For this review, take the finished solid that the model builds, in its own axes (mm). Face numbers are marked on the shaded views. Coordinates: 2 decimals unless noted, no trailing zeros. Write each loop counter-clockwise with the first axis right and the second up, starting at its lowest first coordinate (ties: lowest second). Pieces come first, ordered by that corner, then holes. Notation, with made-up numbers: (77, 75) - (107, 75) arc R27 cw to (107, 111) - close; hole circle Ø10 at (19.25, 68.25). An arc over 180 degrees is marked (long way). Use one line per item in the form item = value. Start each with the question number.
1) Mouldability with a two-part tool opening along X and no side actions: class the marked faces 1 and 2 as pulls with the +X half, pulls with the -X half, needs draft (parallel to the pull), parting line crosses it, or undercut.
2) Insertion check: P1, Ø1, axis at y = -14.5, z = 17, coming from the -X side; P2, Ø1.5, axis at x = 2, z = 4.5, coming from the +Y side; P3, Ø3, axis at x = -110, y = 18.5, coming from the +Z side. Each pin has a flat end and moves straight along its axis. Give the tip position at first contact, or say it passes through.
3) We need section A-A (z = 20.5). Give the boundary of the cut face in (x, y), plus the area to 3 significant figures.
4) We need section B-B (x = -24). Give the boundary of the cut face in (y, z), plus the area to 3 significant figures.
5) For L1, parallel to Y at x = -130.25, z = 0; L2, parallel to Y at x = -147, z = 0; L3, parallel to X at y = -14.5, z = -16.5, list the stretches that pass through material, from the lowest coordinate up. Write a range as from..to.
```python
from build123d import *

# Parameters (mm, degrees)
BOSS_EXTRUDE1_START      = 80
SKETCH2_R                = 17.5
BOSS_EXTRUDE1_DEPTH      = 80
BOSS_EXTRUDE2_REACH      = 163.943
BOSS_EXTRUDE2_END_RADIUS = 17.5
SKETCH4_R                = 17.5
BOSS_EXTRUDE3_DEPTH      = 5
HOLE1_D                  = 10.106
HOLE1_DEPTH              = 37.5
HOLE1_CBORE_D            = 13
HOLE1_CBORE_DEPTH        = 9.5
HOLE1_TIP                = 2.91735091
CHAMFER1_SIZE            = 2.55
CHAMFER2_SIZE            = 2


with BuildPart() as part:
    # Sketch1 → Revolve1 (revolve)
    with BuildSketch(Plane.XY, mode=Mode.PRIVATE) as revolve1_sk:
        Polygon((-74.5, 22.5), (-74.5, 0), (74.5, 0), (74.5, 22.5), (70, 22.5), (70, 17.5), (-70, 17.5), (-70, 22.5), align=None)
    revolve(revolve1_sk.sketch.rotate(Axis((-74.5, 0, 0), (1, 0, 0)), 270), axis=Axis((-74.5, 0, 0), (1, 0, 0)))

    # Sketch2 → Boss-Extrude1 (add)
    with BuildSketch(Plane.ZY.offset(74.5).offset(BOSS_EXTRUDE1_START)):
        with Locations(Location((0, 0, 0), (0, 0, 180))):
            Circle(SKETCH2_R)
    extrude(amount=-BOSS_EXTRUDE1_DEPTH)

    # Boss-Extrude2: up to this cylinder (the profile starts outside it)
    boss_extrude2_end = Plane(origin=(-114.5, 0, 0), z_dir=(1, 0, 0)) * Cylinder(BOSS_EXTRUDE2_END_RADIUS, 363.886, mode=Mode.PRIVATE)
    # Sketch3 → Boss-Extrude2 (add, up to the surface)
    with BuildSketch(Plane(origin=(0, 20.5, 0), x_dir=(1, 0, 0), z_dir=(0, 1, 0)), mode=Mode.PRIVATE) as boss_extrude2_sk1:
        with BuildLine():
            Line((-134.5, -5), (-94.5, -5))
            ThreePointArc((-94.5, -5), (-89.5, 0), (-94.5, 5))
            Line((-94.5, 5), (-134.5, 5))
            ThreePointArc((-134.5, 5), (-139.5, 0), (-134.5, -5))
        make_face()
    boss_extrude2_tool1 = extrude(boss_extrude2_sk1.sketch, amount=-BOSS_EXTRUDE2_REACH, mode=Mode.PRIVATE) - boss_extrude2_end
    add(boss_extrude2_tool1.solids().sort_by_distance((-114.5, 20.5, 0))[0])

    # Sketch4 → Boss-Extrude3 (add)
    with BuildSketch(Plane(origin=(74.5, 0, 0), x_dir=(0, 0, -1), z_dir=(1, 0, 0))):
        Circle(SKETCH4_R)
    extrude(amount=BOSS_EXTRUDE3_DEPTH)

    # Hole1
    with Locations(Plane.ZY.offset(154.5)):
        with Locations((0, 0)):
            CounterBoreHole(HOLE1_D / 2, HOLE1_CBORE_D / 2, HOLE1_CBORE_DEPTH, depth=HOLE1_DEPTH)
            with Locations((0, 0, -(HOLE1_DEPTH + HOLE1_TIP / 2))):  # 120° drill point
                Cone(0, HOLE1_D / 2, HOLE1_TIP, mode=Mode.SUBTRACT)

    # Chamfer1
    chamfer1_edges = [part.edges().sort_by_distance(p)[0] for p in [
        (-154.5, 0, -6.5),
    ]]
    chamfer(chamfer1_edges, length=CHAMFER1_SIZE)

    # Chamfer2
    chamfer2_edges = [part.edges().sort_by_distance(p)[0] for p in [
        (-154.5, 0, 17.5),
    ]]
    chamfer(chamfer2_edges, length=CHAMFER2_SIZE)


solid = part.part
```
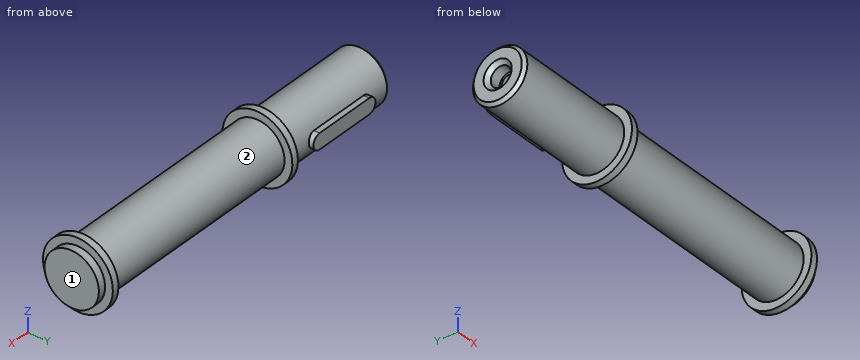
Determined:
q1.face_1 = pulls with the +X half
q1.face_2 = undercut
q2.P1 = -74.5
q2.P2 = 17.09
q2.P3 = 5
q3.outline = (-74.5, -9.27) - (-70, -9.27) - (-70, 9.27) - (-74.5, 9.27) - close; (70, -9.27) - (74.5, -9.27) - (74.5, 9.27) - (70, 9.27) - close
q3.area = 167 mm²
q4.outline = circle Ø35 at (0, 0)
q4.area = 962 mm²
q5.L1 = -17.5..-5.05, 5.05..20.5
q5.L2 = -17.5..-6.5, 6.5..17.5
q5.L3 = -74.5..-70, 70..74.5
